```python
from build123d import *

# Parameters (mm, degrees)
SKETCH1_W           = 42
SKETCH1_H           = 42
BOSS_EXTRUDE2_DEPTH = 48
SKETCH5_R           = 11
BOSS_EXTRUDE3_DEPTH = 2
SKETCH6_R           = 2.5
BOSS_EXTRUDE4_DEPTH = 22


with BuildPart() as part:
    # Sketch1 → Boss-Extrude2 (new body)
    with BuildSketch(Plane(origin=(0, 0, 0), x_dir=(1, 0, 0), z_dir=(0, 1, 0))):
        Rectangle(SKETCH1_W, SKETCH1_H)
    extrude(amount=-BOSS_EXTRUDE2_DEPTH)

    # Sketch5 → Boss-Extrude3 (add)
    with BuildSketch(Plane(origin=(0, 0, 0), x_dir=(1, 0, 0), z_dir=(0, 1, 0))):
        with Locations(Location((0, 0, 0), (0, 0, 270))):
            Circle(SKETCH5_R)
    extrude(amount=BOSS_EXTRUDE3_DEPTH)

    # Sketch6 → Boss-Extrude4 (add)
    with BuildSketch(Plane(origin=(0, 2, 0), x_dir=(1, 0, 0), z_dir=(0, 1, 0))):
        with Locations(Location((0, 0, 0), (0, 0, 270))):
            Circle(SKETCH6_R)
    extrude(amount=BOSS_EXTRUDE4_DEPTH)


solid = part.part
```
The model under review builds one solid part; all positions refer to its coordinate system, in mm. A direction names the side the tool comes from. Round coordinates to 2 decimals unless told otherwise and drop trailing zeros. Order: outer loops, then holes, each group sorted by start corner. A loop starts at its lowest first (then second) coordinate and runs counter-clockwise, first axis right, second up.
(1) Take a section at C-C, the plane y = 6.5. State the section outline as (x, z) points, plus the area to 3 significant figures.
Working result:
outline: circle Ø5 at (0, 0)
area: 19.6 mm2
(2) Wall thickness on L1, parallel to Y at x = -18.5, z = 0; L2, parallel to Y at x = 0.5, z = 8; L3, parallel to Z at x = -1, y = 5: over which ranges is each line inside the solid? List them lowest first.
Working result:
L1: y = -48 to 0
L2: y = -48 to 2
L3: z = -2.29 to 2.29
(3) Take a section at A-A, the plane z = 0. State the section outline as (x, y) points.
Working result:
outline: (-21, -48) - (21, -48) - (21, 0) - (11, 0) - (11, 2) - (2.5, 2) - (2.5, 24) - (-2.5, 24) - (-2.5, 2) - (-11, 2) - (-11, 0) - (-21, 0) - close
(4) Take a section at D-D, the plane x = -6.5. State the section outline as (y, z) points, plus the area to 3 significant figures.
Working result:
outline: (-48, -21) - (0, -21) - (0, -8.87) - (2, -8.87) - (2, 8.87) - (0, 8.87) - (0, 21) - (-48, 21) - close
area: 2,050 mm2
(5) Tool access review of faces 1 (the face through (0, -48, 0)), 2 (the face through (-10, 0, -10)): name each direction out of +Z, -Z, +X, -X, +Y, -Y from which nothing blocks a thin tool from reaching the whole face with its end or side.
Working result:
face 1: +Z, -Z, +X, -X, -Y
face 2: +Y
(6) Take a section at B-B, the plane x = 0. State the section outline as (y, z) points.
Working result:
outline: (-48, -21) - (0, -21) - (0, -11) - (2, -11) - (2, -2.5) - (24, -2.5) - (24, 2.5) - (2, 2.5) - (2, 11) - (0, 11) - (0, 21) - (-48, 21) - close
